Solid Edge part; units mm, degrees
sketch "Sketch1" plane through (0, 0, 0) normal (0, 0, 1) x (1, 0, 0)
  line L0 (-50, -25) -> (50, -25)
  line L1 (50, -25) -> (50, 25)
  line L2 (50, 25) -> (-50, 25)
  line L3 (-50, 25) -> (-50, -25)
extrude "Protrusion1" add sketch "Sketch1" along normal blind 10
chamfer "Fase" distance 1 angle 45 4 edges at (0, -25, 10) (50, 0, 10) (0, 25, 10) (-50, 0, 10)
hole "Hole1" at (37.9, 19, 10) direction (0, 0, -1) diameter 4.5 depth 8
hole "Hole2" at (37.9, -6, 10) direction (0, 0, -1) diameter 4.5 depth 8
hole "Hole3" at (-37.9, -6, 10) direction (0, 0, -1) diameter 4.5 depth 8
hole "Hole4" at (-37.9, 19, 10) direction (0, 0, -1) diameter 4.5 depth 8
Model file for the job. Use its own axes, mm. A direction names the side the tool comes from. Coordinates: 2 decimals unless noted, no trailing zeros. Loops run counter-clockwise (first coordinate to the right, second up) from the corner with the lowest first, then second, coordinate; pieces in that order, holes last. Notation, with made-up numbers: (-10.5, -32) - (35.5, -32) arc R28 cw to (35.5, -6) - close; hole circle Ø6 at (59.25, -37.5). An arc over 180 degrees is marked (long way). Write item = value, one per line. Start each with the question number.
Item 1: Saw through at B-B, the plane y = 19. List the corners of the cut face in (x, z).
Item 2: 3-axis set-ups, long thin cutter, end or side, ignore diameter. For faces 1 (the face through (50, 0, 4)), 2 (the face through (36.003, 17.79, 5.944)): which of +Z, -Z, +X, -X, +Y, -Y reach the whole face in a straight line?
Item 3: Wall check: probe 1 along Y at (x, z) = (-37.9, 7.5); probe 2 along X at (y, z) = (19, 5.5); probe 3 along Y at (x, z) = (-37, 3.5). Give the ranges that are in metal, low to high. Write a range as [from, to].
Item 4: Drop flat-ended pins along their axis: pin 1 Ø6 at (x, y) = (37.9, 19) entering from +Z; pin 2 Ø1.3 at (x, y) = (37.5, 19.5) entering from +Z. Give the stop position or say it passes through.
Item 5: Pull direction Y, two halves, no side cores. Call faces 3 (the face through (-38, 19, 2)), 4 (the face through (-35.904, -7.038, 5.944)), 5 (the face through (1, 25, 4)), 6 (the face through (-1, 0, 10)): +Y half, -Y half, draft (parallel to the pull), parting line (faces both ways), or undercut.
Item 6: Saw through at A-A, the plane x = 37.9. List the corners of the cut face in (y, z), then the cut area to 3 significant figures.
Answers:
q1.outline = (-50, 0) - (50, 0) - (50, 9) - (49, 10) - (40.15, 10) - (40.15, 2) - (35.65, 2) - (35.65, 10) - (-35.65, 10) - (-35.65, 2) - (-40.15, 2) - (-40.15, 10) - (-49, 10) - (-50, 9) - close
q2.face_1 = +Z, -Z, +X, +Y, -Y
q2.face_2 = +Z
q3.probe_1 = [-25, -8.25], [-3.75, 16.75], [21.25, 25]
q3.probe_2 = [-50, -40.15], [-35.65, 35.65], [40.15, 50]
q3.probe_3 = [-25, -8.06], [-3.94, 16.94], [21.06, 25]
q4.pin_1 = 10
q4.pin_2 = 2
q5.face_3 = undercut
q5.face_4 = undercut
q5.face_5 = +Y half
q5.face_6 = draft
q6.outline = (-25, 0) - (25, 0) - (25, 9) - (24, 10) - (21.25, 10) - (21.25, 2) - (16.75, 2) - (16.75, 10) - (-3.75, 10) - (-3.75, 2) - (-8.25, 2) - (-8.25, 10) - (-24, 10) - (-25, 9) - close
q6.area = 427 mm2
